Read the model definition and answer for the solid it produces. Units are mm, in the model's axes. Round coordinates to 2 decimals unless told otherwise and drop trailing zeros. Loops run counter-clockwise (first coordinate to the right, second up) from the corner with the lowest first, then second, coordinate; pieces in that order, holes last. Notation, with made-up numbers: (-36, 87.25) -> (-30, 87.25) arc R18 ccw to (-30, 99.25) -> close; hole circle Ø4 at (-7.75, -8.5). An arc over 180 degrees is marked (long way). Put each result on its own line as item: value.
from build123d import *

# Parameters (mm, degrees)
F1_DEPTH = 25.4
F2_R     = 5.08
F3_R     = 5.08
F4_R     = 5.08
F6_DEPTH = 41.656


with BuildPart() as f1:
    # F0 (on Top) → F1 (new body)
    with BuildSketch(Plane.XY):
        Polygon((0, 38.1), (0, 0), (63.5, 0), (63.5, 38.1), (50.8, 38.1), (12.7, 38.1), align=None)
    extrude(amount=F1_DEPTH)

    # F2
    f2_edges = [f1.edges().sort_by_distance(p)[0] for p in [
        (0, 0, 12.7),
    ]]
    fillet(f2_edges, radius=F2_R)

    # F3
    f3_edges = [f1.edges().sort_by_distance(p)[0] for p in [
        (1.487898, 1.487898, 25.4),
    ]]
    fillet(f3_edges, radius=F3_R)

    # F4
    f4_edges = [f1.edges().sort_by_distance(p)[0] for p in [
        (34.29, 38.1, 25.4),
    ]]
    fillet(f4_edges, radius=F4_R)

    # F5 (on face) → F6 (cut)
    with BuildSketch(Plane.XZ):
        with BuildLine():
            Line((63.5, 20.32), (36.6062117726, 20.32))
            ThreePointArc((36.6062117726, 20.32), (44.8198393028, 3.2603855953), (63.5, 6.35))
            Line((63.5, 6.35), (63.5, 20.32))
        make_face()
    extrude(amount=-F6_DEPTH, mode=Mode.SUBTRACT)


solid = f1.part
Item 1: A flat-ended cylindrical pin translates along its axis: pin 1 Ø5 at (y, z) = (10, 12) entering from +X. Find the tip coordinate at first contact, or state that the pin passes through.
Derived:
pin 1: stops at x = 38.35
Item 2: The part is cut by section B-B (z = 3). Determine the outline of the cut face in (x, y), then the cut area to 3 significant figures.
Derived:
outline: (0, 5.08) arc R5.08 ccw to (5.08, 0) -> (45.34, 0) -> (45.34, 38.1) -> (5.08, 38.1) arc R5.08 ccw to (0, 33.02) -> close; (58.85, 0) -> (63.5, 0) -> (63.5, 38.1) -> (58.85, 38.1) -> close
area: 1,890 mm^2
Item 3: The part is cut by section A-A (x = 54.5). Determine the outline of the cut face in (y, z).
Derived:
outline: (0, 0) -> (38.1, 0) -> (38.1, 1.67) -> (0, 1.67) -> close; (0, 20.32) -> (38.1, 20.32) arc R5.08 ccw to (33.02, 25.4) -> (5.08, 25.4) arc R5.08 ccw to start
Item 4: The part is cut by section C-C (y = 26). Determine the outline of the cut face in (x, z), then the cut area to 3 significant figures.
Derived:
outline: (0, 0) -> (63.5, 0) -> (63.5, 6.35) arc R15.79 cw to (36.61, 20.32) -> (63.5, 20.32) -> (63.5, 25.4) -> (5.08, 25.4) arc R5.08 ccw to (0, 20.32) -> close
area: 1,170 mm^2
Item 5: Find the intervals of material crossed by line 1 along Z through (x, y) = (58, 25); line 2 along Z through (x, y) = (43, 2.5); line 3 along X through (y, z) = (24.5, 17), in increasing order.
Derived:
line 1: z = 0 to 2.63, 20.32 to 25.4
line 2: z = 0 to 4.37, 20.32 to 24.7
line 3: x = 0 to 36.31
Item 6: The part is cut by section D-D (z = 11.5). Determine the outline of the cut face in (x, y).
Derived:
outline: (0, 5.08) arc R5.08 ccw to (5.08, 0) -> (37.4, 0) -> (37.4, 38.1) -> (5.08, 38.1) arc R5.08 ccw to (0, 33.02) -> close
Item 7: For a pull along X with two mould halves and no side action, classify faces 1 (the cylindrical face through (1.449, 1.528, 10.302)), 2 (the cylindrical face through (44.569, 18.783, 3.394)), 3 (the flat face through (50, 19, 20.32)) as pulls with the +X half, pulls with the -X half, needs draft (parallel to the pull), parting line crosses it, or undercut.
Derived:
face 1: pulls with the -X half
face 2: undercut
face 3: needs draft
